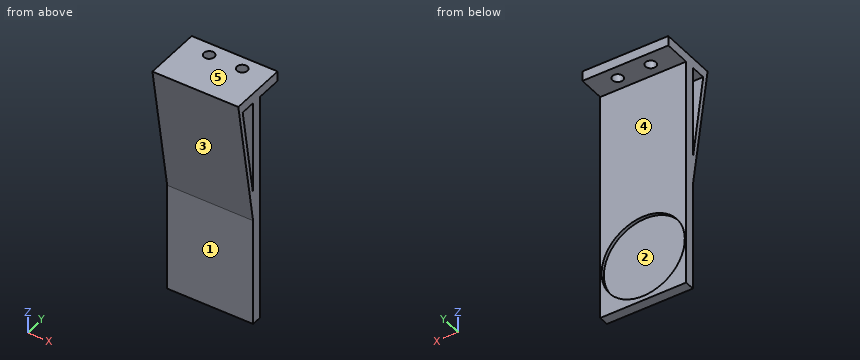
from build123d import *

# Parameters (mm, degrees)
EXTRUDE_1_DEPTH     = 26
SKETCH_2_R          = 1.6
CUT_EXTRUDE_1_DEPTH = 10
SKETCH_3_R          = 12.6
CUT_EXTRUDE_2_DEPTH = 1


with BuildPart() as part:
    # 草图1 → 凸台-拉伸1 (new body)
    with BuildSketch(Plane(origin=(0, 0, 0), x_dir=(0, 0, -1), z_dir=(1, 0, 0))):
        Polygon((-36.5, -8.11923054), (3.755241517, -1.5), (36.5, -1.5), (36.5, 1.5), (-33.5, 1.5), (-33.5, 9.5), (-36.5, 9.5), align=None)
        Polygon((-4.861119654, -1.5), (-33.5, -6.160415563), (-33.5, -1.5), align=None, mode=Mode.SUBTRACT)
    extrude(amount=EXTRUDE_1_DEPTH)

    # 草图2 → 切除-拉伸1 (cut)
    with BuildSketch(Plane.XY.offset(36.5)):
        with Locations((8, 5.5)):
            Circle(SKETCH_2_R)
        with Locations((18, 5.5)):
            Circle(SKETCH_2_R)
    extrude(amount=-CUT_EXTRUDE_1_DEPTH, mode=Mode.SUBTRACT)

    # 草图3 → 切除-拉伸2 (cut)
    with BuildSketch(Plane(origin=(0, 1.5, 0), x_dir=(1, 0, 0), z_dir=(0, 1, 0))):
        with Locations(Location((13, 22.563165018, 0), (0, 0, 270))):
            Circle(SKETCH_3_R)
    extrude(amount=-CUT_EXTRUDE_2_DEPTH, mode=Mode.SUBTRACT)


solid = part.part
Here's how the part is built. I have some questions about the finished solid (model axes, mm). Face numbers are marked on the shaded views. A direction names the side the tool comes from. Coordinates: 2 decimals unless noted, no trailing zeros. Order: outer loops, then holes, each group sorted by start corner. A loop starts at its lowest first (then second) coordinate and runs counter-clockwise, first axis right, second up. Notation, with made-up numbers: (-35, 31.5) - (-26, 31.5) arc R34 cw to (-26, 61.5) - close; hole circle Ø4 at (37, 82). An arc over 180 degrees is marked (long way). Use CSV: the item, a comma, the result in double quotes. Start each with the question number.
1. I'm going to push flat-ended pins straight in: pin 1 (10 mm diameter, centred on x = 6.5, z = -8.5, fed in from -Y); pin 2 (6 mm diameter, centred on x = 5, y = -2, fed in from -Z); pin 3 (4 mm diameter, centred on x = 5, z = 9.5, fed in from +Y); pin 4 (4 mm diameter, centred on x = 16, z = 17.5, fed in from -Y). Where does each tip first touch, or does it pass through?
2. If we mould it in two halves opening along Z, with no side actions, what happens to the marked faces 1, 2 and 3? For each: +Z half, -Z half, draft (parallel to the pull), parting line (faces both ways), or undercut.
3. Suppose I cut it at C-C on y = -3.5. List the corners of the cut face in (x, z) for me.
4. Please list where these lines run through material, in increasing order: line 1 (Y direction, x = 3.5, z = -9.5); line 2 (Y direction, x = 4, z = -31); line 3 (Y direction, x = 8, z = 35.75). Write a range as from..to.
5. Suppose I cut it at A-A on y = 5.5. List the corners of the cut face in (x, z) for me, then the cut area to 3 significant figures.
6. Suppose I cut it at B-B on x = 13. List the corners of the cut face in (y, z) for me, then the cut area to 3 significant figures.
7. Suppose I cut it at D-D on z = 10. List the corners of the cut face in (x, y) for me.
8. For the marked faces 4 and 5, which set-ups out of +Z, -Z, +X, -X, +Y, -Y let a thin tool reach every point of the face, with its end or its side?
Output:
1,pin 1,"stops at y = -1.54"
1,pin 2,"stops at z = -36.5"
1,pin 3,"stops at y = 1.5"
1,pin 4,"stops at y = -5.32"
2,face 1,"draft"
2,face 2,"undercut"
2,face 3,"-Z half"
3,outline,"(0, 8.41) - (26, 8.41) - (26, 17.15) - (0, 17.15) - close; (0, 33.5) - (26, 33.5) - (26, 36.5) - (0, 36.5) - close"
4,line 1,"y = -1.5..1.5"
4,line 2,"y = -1.5..0.5"
4,line 3,"y = -8..3.9, 7.1..9.5"
5,outline,"(0, 33.5) - (6.4, 33.5) - (6.4, 36.5) - (0, 36.5) - close; (9.6, 33.5) - (16.4, 33.5) - (16.4, 36.5) - (9.6, 36.5) - close; (19.6, 33.5) - (26, 33.5) - (26, 36.5) - (19.6, 36.5) - close"
5,area,"58.8 mm2"
6,outline,"(-8.12, 36.5) - (-1.5, -3.76) - (-1.5, -36.5) - (1.5, -36.5) - (1.5, -35.16) - (0.5, -35.16) - (0.5, -9.96) - (1.5, -9.96) - (1.5, 33.5) - (9.5, 33.5) - (9.5, 36.5) - close; hole (-6.16, 33.5) - (-1.5, 4.86) - (-1.5, 33.5) - close"
6,area,"284 mm2"
7,outline,"(0, -3.76) - (26, -3.76) - (26, -2.34) - (0, -2.34) - close; (0, -1.5) - (26, -1.5) - (26, 1.5) - (0, 1.5) - close"
8,face 4,"-Z, +X, -X, +Y"
8,face 5,"+Z, +X, -X, +Y, -Y"
